Could you check a few things on this model? Use its own coordinates, in mm. Coordinates: 2 decimals unless noted, no trailing zeros. Loops run counter-clockwise (first coordinate to the right, second up) from the corner with the lowest first, then second, coordinate; pieces in that order, holes last.
from build123d import *

# Parameters (mm, degrees)
BOSS_EXTRUDE1_DEPTH = 10.16
SKETCH2_W           = 10.166490401
SKETCH2_H           = 81.316938585
SKETCH2_W_2         = 10.166490402
SKETCH2_H_2         = 81.316938584
SKETCH2_W_3         = 82.271298803
SKETCH2_H_3         = 10.16
CUT_EXTRUDE2_DEPTH  = 137.414
CUT_EXTRUDE3_DEPTH  = 1426.179737238
SKETCH5_W           = 82.296
SKETCH5_H           = 10.16
CUT_EXTRUDE4_DEPTH  = 1408.779997291
CUT_EXTRUDE5_DEPTH  = 1408.779997291
CUT_EXTRUDE6_DEPTH  = 25.4


with BuildPart() as part:
    # Sketch1 → Boss-Extrude1 (new body)
    with BuildSketch(Plane.XY):
        with BuildLine():
            Line((0, 0), (1345.447057269, 0))
            Line((1345.447057269, 0), (1156.937235756, -454.288839135))
            add(Edge.make_bspline(
                [(1156.937235756, -454.288839135), (1155.965204773, -456.631331547), (1154.630956054, -458.816896883), (1152.225947859, -461.69350105), (1151.355065983, -462.590813772), (1149.473312624, -464.260936999), (1148.45987476, -465.033112958), (1146.360299176, -466.401155283), (1145.26635201, -467.004685932), (1142.990856866, -468.052074807), (1141.798989191, -468.498505895), (1138.174492983, -469.560599459), (1135.699262078, -469.911644948), (1133.16419506, -469.9)],
                knots=[0, 0, 0, 0, 0.25, 0.25, 0.375, 0.375, 0.5, 0.5, 0.625, 0.625, 0.75, 0.75, 1, 1, 1, 1], degree=3))
            Line((1133.16419506, -469.9), (212.282862208, -469.9))
            add(Edge.make_bspline(
                [(188.509821513, -454.288839135), (189.481852496, -456.631331547), (190.816101215, -458.816896883), (193.22110941, -461.69350105), (194.091991286, -462.590813772), (195.973744645, -464.260936999), (196.987182509, -465.033112958), (199.086758093, -466.401155283), (200.180705259, -467.004685932), (202.456200403, -468.052074807), (203.648068078, -468.498505895), (207.272564286, -469.560599459), (209.747795191, -469.911644948), (212.282862208, -469.9)],
                knots=[0, 0, 0, 0, 0.25, 0.25, 0.375, 0.375, 0.5, 0.5, 0.625, 0.625, 0.75, 0.75, 1, 1, 1, 1], degree=3))
            Line((188.509821513, -454.288839135), (0, 0))
        make_face()
    extrude(amount=BOSS_EXTRUDE1_DEPTH)

    # Sketch2 → Cut-Extrude2 (cut)
    with BuildSketch(Plane.XY.offset(10.16)):
        with Locations((461.924984631, -337.764592123)):
            Rectangle(SKETCH2_W, SKETCH2_H)
        with Locations((883.522072638, -337.764592123)):
            Rectangle(SKETCH2_W_2, SKETCH2_H)
        with Locations((883.522072638, -175.130714953)):
            Rectangle(SKETCH2_W_2, SKETCH2_H_2)
        with Locations((461.924984631, -175.130714953)):
            Rectangle(SKETCH2_W, SKETCH2_H_2)
        with Locations((837.303178036, -464.82)):
            Rectangle(SKETCH2_W_3, SKETCH2_H_3)
        with Locations((672.723528635, -464.82)):
            Rectangle(SKETCH2_W_3, SKETCH2_H_3)
        with Locations((508.143879233, -464.82)):
            Rectangle(SKETCH2_W_3, SKETCH2_H_3)
    extrude(amount=-CUT_EXTRUDE2_DEPTH, mode=Mode.SUBTRACT)

    # Sketch4 → Cut-Extrude3 (cut, through all)
    with BuildSketch(Plane.XY.offset(10.16)):
        Polygon((0, 0), (1345.447057269, 0), (1327.002268746, -44.45), (18.444788523, -44.45), align=None)
    extrude(amount=-CUT_EXTRUDE3_DEPTH, mode=Mode.SUBTRACT)

    # Sketch5 → Cut-Extrude4 (cut, through all)
    with BuildSketch(Plane.XY.offset(10.16)):
        with Locations((508.131528634, -49.53)):
            Rectangle(SKETCH5_W, SKETCH5_H)
        with Locations((672.723528634, -49.53)):
            Rectangle(SKETCH5_W, SKETCH5_H)
        with Locations((837.315528634, -49.53)):
            Rectangle(SKETCH5_W, SKETCH5_H)
    extrude(amount=-CUT_EXTRUDE4_DEPTH, mode=Mode.SUBTRACT)

    # Sketch6 → Cut-Extrude5 (cut, through all)
    with BuildSketch(Plane.XY.offset(10.16)):
        Polygon((192.807539001, -448.077869782), (224.982862208, -469.9), (232.080223429, -549.766419732), (-59.510742861, -242.335130221), (-120.238907144, 37.382474964), (56.544788523, -44.45), (56.544788523, -119.698975594), align=None)
        Polygon((1120.46419506, -469.9), (1113.36683384, -549.766419732), (1404.95780013, -242.335130221), (1465.685964413, 37.382474964), (1288.902268746, -44.45), (1288.902268746, -119.698975594), (1152.639518267, -448.077869782), align=None)
    extrude(amount=-CUT_EXTRUDE5_DEPTH, mode=Mode.SUBTRACT)

    # Sketch7 → Cut-Extrude6 (cut)
    with BuildSketch(Plane.XY.offset(10.16)):
        with BuildLine():
            Line((301.182862208, -469.9), (-145.537284928, -469.9))
            Line((-145.537284928, -469.9), (-145.537284928, 127.88628448))
            Line((-145.537284928, 127.88628448), (224.982862208, 127.88628448))
            Line((224.982862208, 127.88628448), (224.982862208, -393.7))
            ThreePointArc((224.982862208, -393.7), (247.301325482, -447.581536726), (301.182862208, -469.9))
        make_face()
        with BuildLine():
            Line((1044.26419506, -469.9), (1351.858793672, -469.9))
            Line((1351.858793672, -469.9), (1351.858793672, 23.69842382))
            Line((1351.858793672, 23.69842382), (1120.46419506, 23.69842382))
            Line((1120.46419506, 23.69842382), (1120.46419506, -393.7))
            ThreePointArc((1120.46419506, -393.7), (1098.145731787, -447.581536726), (1044.26419506, -469.9))
        make_face()
    extrude(amount=-CUT_EXTRUDE6_DEPTH, mode=Mode.SUBTRACT)


solid = part.part
(1) Imagine slicing it at B-B, the plane x = 484.5. Write out the boundary of the cut face in (y, z).
Answers:
outline: (-459.74, 0) - (-54.61, 0) - (-54.61, 10.16) - (-459.74, 10.16) - close
(2) Imagine slicing it at D-D, the plane y = -431.5. Write out the boundary of the cut face in (x, z), and give its area (3 significant figures).
Answers:
outline: (235.02, 0) - (1110.43, 0) - (1110.43, 10.16) - (235.02, 10.16) - close
area: 8,890 mm2
(3) I need wall thicknesses on probe 1 along X at (y, z) = (-314, 4); probe 2 along Y at (x, z) = (689, 4.5); probe 3 along X at (y, z) = (-423, 5.25). Which ranges of each line are inside material? Lowest first, please.
Answers:
probe 1: x = 224.98 to 456.84, 467.01 to 878.44, 888.61 to 1120.46
probe 2: y = -459.74 to -54.61
probe 3: x = 230.84 to 1114.61
(4) For pin 1 (1.5 mm diameter, centred on x = 705, z = 7, fed in from +Y); pin 2 (5 mm diameter, centred on y = -466.5, z = 7, fed in from +X); pin 3 (2 mm diameter, centred on y = -426.5, z = 5.5, fed in from -X), each with a flat end and sliding along its axis, tell me the tip position at first contact or that it passes through.
Answers:
pin 1: stops at y = -54.61
pin 2: stops at x = 1073.66
pin 3: stops at x = 231.94
(5) Imagine slicing it at A-A, the plane y = -159.5. Write out the boundary of the cut face in (x, z), and give its area (3 significant figures).
Answers:
outline: (224.98, 0) - (456.84, 0) - (456.84, 10.16) - (224.98, 10.16) - close; (467.01, 0) - (878.44, 0) - (878.44, 10.16) - (467.01, 10.16) - close; (888.61, 0) - (1120.46, 0) - (1120.46, 10.16) - (888.61, 10.16) - close
area: 8,890 mm2
(6) Imagine slicing it at C-C, the plane z = 6.5. State how many separate pieces and enclosed holes the cut face has, and give its area (3 significant figures).
Answers:
separate pieces: 1
enclosed holes: 4
area: 370,000 mm2
